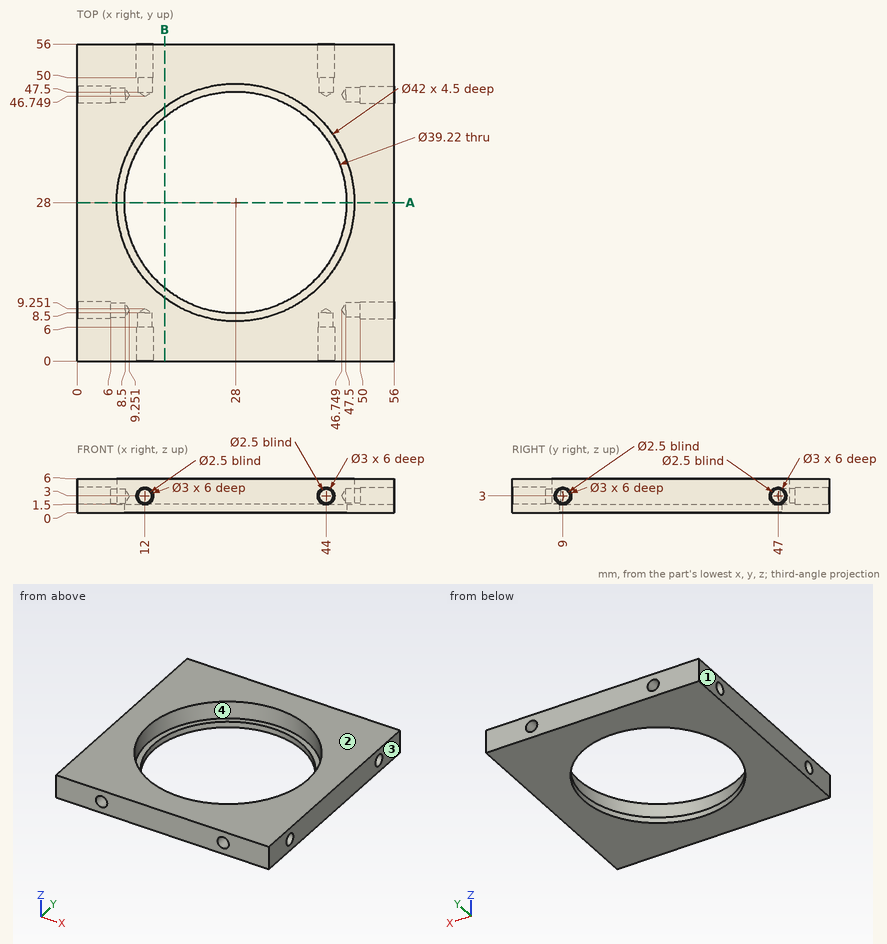
Source: three-view drawing plus pictorial views. Frame: mm from the lowest corner of the part. Round coordinates to 2 decimals unless told otherwise and drop trailing zeros. Loops run counter-clockwise (first coordinate to the right, second up) from the corner with the lowest first, then second, coordinate; pieces in that order, holes last.
Q1. First-contact query: P1, Ø0.9, axis at y = 46.5, z = 2.5, coming from the -X side; P2, Ø1.5, axis at y = 38, z = 4.5, coming from the -X side; P3, Ø2, axis at x = 44, z = 3, coming from the -Y side; P4, Ø2, axis at y = 47, z = 3, coming from the +X side. Flat tips, straight axial feed; report the tip coordinate or a pass-through.
Q2. Section A-A, the plane y = 28. Return loops of the section in (x, z).
Q3. Ray query, line 1 (Y direction, x = 3.45, z = 3); line 2 (X direction, y = 51.5, z = 3.2); line 3 (Z direction, x = 49.15, y = 47). Return the intervals inside material, ascending.
Q4. Mould query, pull axis X, two halves, no side actions, for the marked faces 1, 2, 3 and 4. Classes: pulls with the +X half, pulls with the -X half, needs draft (parallel to the pull), parting line crosses it, or undercut.
Q5. Section B-B, the plane x = 15.5. Return loops of the section in (y, z).
Solutions:
1. P1: stops at x = 8.56
1. P2: stops at x = 0
1. P3: stops at y = 8.65
1. P4: stops at x = 47.35
2. outline: (0, 0) - (8.39, 0) - (8.39, 1.5) - (7, 1.5) - (7, 6) - (0, 6) - close; (47.61, 0) - (56, 0) - (56, 6) - (49, 6) - (49, 1.5) - (47.61, 1.5) - close
3. line 1: y = 0 to 7.5, 10.5 to 45.5, 48.5 to 56
3. line 2: x = 0 to 10.51, 13.49 to 42.51, 45.49 to 56
3. line 3: z = 0 to 1.75, 4.25 to 6
4. face 1: pulls with the -X half
4. face 2: needs draft
4. face 3: pulls with the +X half
4. face 4: undercut
5. outline: (0, 0) - (12.89, 0) - (12.89, 1.5) - (11.13, 1.5) - (11.13, 6) - (0, 6) - close; (43.11, 0) - (56, 0) - (56, 6) - (44.87, 6) - (44.87, 1.5) - (43.11, 1.5) - close
